from build123d import *

# Parameters (mm, degrees)
SKETCH1_W                  = 80.3
SKETCH1_H                  = 66
BOSS_EXTRUDE1_DEPTH        = 2
F_3_2_3_2_DIAMETER_HOLE1_D = 3.2
FILLET1_R                  = 3
SKETCH4_W                  = 75
SKETCH4_H                  = 60.5
CUT_EXTRUDE1_DEPTH         = 3


with BuildPart() as part:
    # Sketch1 → Boss-Extrude1 (new body)
    with BuildSketch(Plane.XY):
        with Locations((40.15, 33)):
            Rectangle(SKETCH1_W, SKETCH1_H)
    extrude(amount=BOSS_EXTRUDE1_DEPTH)

    # Ø3.2 (3.2) Diameter Hole1 (through all)
    with Locations(Plane.XY.offset(2)):
        with Locations((7, 59), (73.3, 59), (73.3, 7), (7, 7)):
            Hole(F_3_2_3_2_DIAMETER_HOLE1_D / 2)

    # Fillet1
    fillet1_edges = [part.edges().sort_by_distance(p)[0] for p in [
        (0, 66, 1),
        (80.3, 66, 1),
        (80.3, 0, 1),
        (0, 0, 1),
    ]]
    fillet(fillet1_edges, radius=FILLET1_R)

    # Sketch4 → Cut-Extrude1 (cut, through all)
    with BuildSketch(Plane.XY.offset(2)):
        with Locations((40.15, 33)):
            Rectangle(SKETCH4_W, SKETCH4_H)
    extrude(amount=-CUT_EXTRUDE1_DEPTH, mode=Mode.SUBTRACT)


solid = part.part
Input: part model. Units: mm. Frame: model coordinates. A direction names the side the tool comes from. Round coordinates to 2 decimals unless told otherwise and drop trailing zeros. Loops run counter-clockwise (first coordinate to the right, second up) from the corner with the lowest first, then second, coordinate; pieces in that order, holes last. Notation, with made-up numbers: (78, 10) -> (118, 10) arc R22 ccw to (118, 41) -> close; hole circle Ø4 at (67, 47.5). An arc over 180 degrees is marked (long way). Answer as a JSON object with one key per item and string values. Group by question number.
1) Section query C-C on y = 30. Output: boundary loops of the cut face in (x, z), plus the area to 3 significant figures.
2) Section query B-B on z = 1. Output: boundary loops of the cut face in (x, y), plus the area to 3 significant figures.
3) Reachability of faces 1 (the flat face through (0, 33, 1)), 2 (the flat face through (40, 63.25, 1)) from +Z, -Z, +X, -X, +Y, -Y: full face, straight path, thin tool, end or side. Return the list, or none.
4) Section query A-A on x = 11. Output: boundary loops of the cut face in (y, z), plus the area to 3 significant figures.
5) Pin query (flat end, axial travel): pin 1 (10 mm diameter, centred on x = 13.5, y = 8.5, fed in from -Z). Return the tip coordinate at first contact, or that it passes through.
6) Ray query, L1, parallel to Y at x = 27.5, z = 0.7; L2, parallel to X at y = 4, z = 0.2. Return the intervals inside material, ascending.
Reply:
{
 "1": {"outline": "(0, 0) -> (2.65, 0) -> (2.65, 2) -> (0, 2) -> close; (77.65, 0) -> (80.3, 0) -> (80.3, 2) -> (77.65, 2) -> close", "area": "10.6 mm2"},
 "2": {"outline": "(0, 3) arc R3 ccw to (3, 0) -> (77.3, 0) arc R3 ccw to (80.3, 3) -> (80.3, 63) arc R3 ccw to (77.3, 66) -> (3, 66) arc R3 ccw to (0, 63) -> close; hole (2.65, 2.75) -> (77.65, 2.75) -> (77.65, 63.25) -> (2.65, 63.25) -> close", "area": "755 mm2"},
 "3": {"face 1": "+Z, -Z, -X, +Y, -Y", "face 2": "+Z, -Z"},
 "4": {"outline": "(0, 0) -> (2.75, 0) -> (2.75, 2) -> (0, 2) -> close; (63.25, 0) -> (66, 0) -> (66, 2) -> (63.25, 2) -> close", "area": "11.0 mm2"},
 "5": {"pin 1": "passes through"},
 "6": {"L1": "y = 0 to 2.75, 63.25 to 66", "L2": "x = 0 to 2.65, 77.65 to 80.3"}
}
